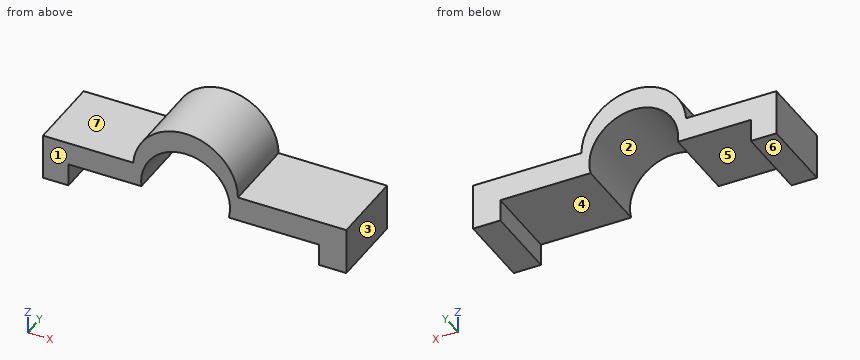
from build123d import *

# Parameters (mm, degrees)
F1_DEPTH = 25


with BuildPart() as f1:
    # F0 (on Front) → F1 (new body)
    with BuildSketch(Plane.XZ):
        with BuildLine():
            Line((50.648533, -37.582681), (50.648533, -44.629429))
            Line((50.648533, -44.629429), (59.456974, -44.629429))
            Line((59.456974, -44.629429), (59.456974, -29.655084))
            Line((59.456974, -29.655084), (24.516825, -29.655084))
            ThreePointArc((24.516825, -29.655084), (8.195501, -12.924194), (-9.248863, -28.480623))
            Line((-9.248863, -28.480623), (-38.316716, -28.480623))
            Line((-38.316716, -28.480623), (-38.316716, -43.161355))
            Line((-38.316716, -43.161355), (-30.095505, -43.161355))
            Line((-30.095505, -43.161355), (-30.095505, -35.820991))
            Line((-30.095505, -35.820991), (-6.60633, -35.820991))
            ThreePointArc((-6.60633, -35.820991), (8.532595, -19.975134), (21.580679, -37.582681))
            Line((21.580679, -37.582681), (50.648533, -37.582681))
        make_face()
    extrude(amount=F1_DEPTH)


solid = f1.part
CAD build for the part. Positions are in the model's coordinates, mm. Face numbers are marked on the shaded views. A direction names the side the tool comes from. Give positions to 0.01 mm unless a question says otherwise; leave off trailing zeros. Write each loop counter-clockwise with the first axis right and the second up, starting at its lowest first coordinate (ties: lowest second). Pieces come first, ordered by that corner, then holes. Notation, with made-up numbers: (-38.75, -39.5) - (-6.75, -39.5) arc R8 cw to (-6.75, -30.5) - close; hole circle Ø9 at (19, 27.25). An arc over 180 degrees is marked (long way). Answer as CSV lines item,"result".
Q1. Band-saw the part on A-A (z = -22.5). Give the cut face in (x, y), and give its area (3 significant figures).
Result set:
outline,"(-7.63, -25) - (-0.52, -25) - (-0.52, 0) - (-7.63, 0) - close; (15.8, -25) - (22.85, -25) - (22.85, 0) - (15.8, 0) - close"
area,"354 mm²"
Q2. Band-saw the part on C-C (x = 38.5). Give the cut face in (y, z), and give its area (3 significant figures).
Result set:
outline,"(-25, -37.58) - (0, -37.58) - (0, -29.66) - (-25, -29.66) - close"
area,"198 mm²"
Q3. Band-saw the part on D-D (z = -16.5). Give the cut face in (x, y).
Result set:
outline,"(-2.8, -25) - (18.02, -25) - (18.02, 0) - (-2.8, 0) - close"
Q4. Pull direction X, two halves, no side cores. Call the marked faces 1, 2, 3 and 4: released by +X, released by -X, zero draft, split by the parting line, or undercut.
Result set:
face 1,"zero draft"
face 2,"undercut"
face 3,"released by +X"
face 4,"undercut"
Q5. Drill centre lines: line 1 (X direction, y = -9.25, z = -40.5); line 2 (Z direction, x = -25, y = -16); line 3 (X direction, y = -8.5, z = -34). Where is each one in solid material? Low to high. Write a range as from..to.
Result set:
line 1,"-38.32..-30.1, 50.65..59.46"
line 2,"-35.82..-28.48"
line 3,"-38.32..-6.69, 21.96..59.46"
Q6. Flat gauge pins, fed straight in: pin 1 Ø7.5 at (x, y) = (35, -18) entering from +Z; pin 2 Ø1.5 at (y, z) = (-12.5, -27.5) entering from -X; pin 3 Ø6 at (x, y) = (-23.5, -20) entering from +Z; pin 4 Ø1 at (x, z) = (-15, -26.5) entering from -Y. Where does each tip first touch, or does it go through?
Result set:
pin 1,"z = -29.66"
pin 2,"x = -9.23"
pin 3,"z = -28.48"
pin 4,"through"
Q7. Band-saw the part on B-B (y = -2). Give the cut face in (x, z).
Result set:
outline,"(-38.32, -43.16) - (-30.1, -43.16) - (-30.1, -35.82) - (-6.61, -35.82) arc R14.33 cw (long way) to (21.58, -37.58) - (50.65, -37.58) - (50.65, -44.63) - (59.46, -44.63) - (59.46, -29.66) - (24.52, -29.66) arc R16.91 ccw to (-9.25, -28.48) - (-38.32, -28.48) - close"
Q8. 3-axis set-ups, long thin cutter, end or side, ignore diameter. For the marked faces 5, 6 and 7: which of +Z, -Z, +X, -X, +Y, -Y reach the whole face in a straight line?
Result set:
face 5,"-Z, +Y, -Y"
face 6,"-Z, -X, +Y, -Y"
face 7,"+Z, -X, +Y, -Y"
